Part model, mm, in its own coordinate system. Face numbers are marked on the shaded views. Give positions to 0.01 mm unless a question says otherwise; leave off trailing zeros. Write each loop counter-clockwise with the first axis right and the second up, starting at its lowest first coordinate (ties: lowest second). Pieces come first, ordered by that corner, then holes.
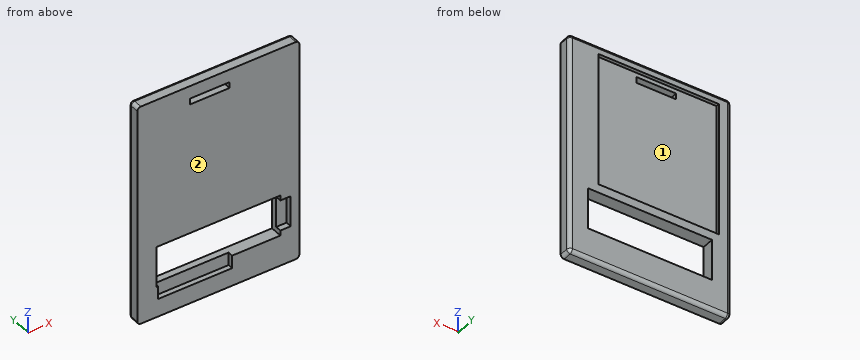
```python
from build123d import *

# Parameters (mm, degrees)
SKETCH1_W           = 94
SKETCH1_H           = 130
BOSS_EXTRUDE1_DEPTH = 7
SKETCH2_W           = 72
SKETCH2_H           = 24
CUT_EXTRUDE1_DEPTH  = 8
SKETCH3_W           = 6
SKETCH3_H           = 18
CUT_EXTRUDE2_DEPTH  = 3.5
SKETCH4_W           = 43
SKETCH4_H           = 7.5
CUT_EXTRUDE3_DEPTH  = 3
SKETCH5_W           = 70
SKETCH5_H           = 78
CUT_EXTRUDE4_DEPTH  = 2
SKETCH6_W           = 23
SKETCH6_H           = 3.5
CUT_EXTRUDE5_DEPTH  = 6
FILLET1_R           = 2


with BuildPart() as part:
    # Sketch1 → Boss-Extrude1 (new body)
    with BuildSketch(Plane(origin=(0, 0, 0), x_dir=(1, 0, 0), z_dir=(0, 1, 0))):
        with Locations((47, 65)):
            Rectangle(SKETCH1_W, SKETCH1_H)
    extrude(amount=BOSS_EXTRUDE1_DEPTH)

    # Sketch2 → Cut-Extrude1 (cut, through all)
    with BuildSketch(Plane(origin=(0, 7, 0), x_dir=(1, 0, 0), z_dir=(0, 1, 0))):
        with Locations((47, 100)):
            Rectangle(SKETCH2_W, SKETCH2_H)
    extrude(amount=-CUT_EXTRUDE1_DEPTH, mode=Mode.SUBTRACT)

    # Sketch3 → Cut-Extrude2 (cut)
    with BuildSketch(Plane.XZ):
        with Locations((86, -100)):
            Rectangle(SKETCH3_W, SKETCH3_H)
    extrude(amount=-CUT_EXTRUDE2_DEPTH, mode=Mode.SUBTRACT)

    # Sketch4 → Cut-Extrude3 (cut)
    with BuildSketch(Plane.XZ):
        with Locations((33.5, -115.75)):
            Rectangle(SKETCH4_W, SKETCH4_H)
    extrude(amount=-CUT_EXTRUDE3_DEPTH, mode=Mode.SUBTRACT)

    # Sketch5 → Cut-Extrude4 (cut)
    with BuildSketch(Plane(origin=(0, 7, 0), x_dir=(1, 0, 0), z_dir=(0, 1, 0))):
        with Locations((42, 44)):
            Rectangle(SKETCH5_W, SKETCH5_H)
    extrude(amount=-CUT_EXTRUDE4_DEPTH, mode=Mode.SUBTRACT)

    # Sketch6 → Cut-Extrude5 (cut, through all)
    with BuildSketch(Plane(origin=(0, 5, 0), x_dir=(1, 0, 0), z_dir=(0, 1, 0))):
        with Locations((42, 9.25)):
            Rectangle(SKETCH6_W, SKETCH6_H)
    extrude(amount=-CUT_EXTRUDE5_DEPTH, mode=Mode.SUBTRACT)

    # Fillet1
    fillet1_edges = [part.edges().sort_by_distance(p)[0] for p in [
        (94, 7, -65),
        (47, 7, -130),
        (0, 7, -65),
        (0, 3.5, -130),
        (94, 3.5, -130),
        (94, 3.5, 0),
        (0, 3.5, 0),
        (47, 7, 0),
    ]]
    fillet(fillet1_edges, radius=FILLET1_R)


solid = part.part
```
1) Saw through at B-B, the plane z = -46. Write the cut outline in (x, y), then the cut area to 3 significant figures.
Answers follow:
outline: (0, 0) - (94, 0) - (94, 5) arc R2 ccw to (92, 7) - (77, 7) - (77, 5) - (7, 5) - (7, 7) - (2, 7) arc R2 ccw to (0, 5) - close
area: 516 mm2
2) Pin check, flat tips, straight feed: pin 1 Ø8 at (x, z) = (33, -114) entering from -Y; pin 2 Ø1.5 at (y, z) = (6, -20) entering from +X; pin 3 Ø1.6 at (y, z) = (6, -48.5) entering from -X; pin 4 Ø5 at (x, z) = (87, -97) entering from -Y. Stop position of each tip, or through.
Answers follow:
pin 1: stops at y = 3
pin 2: stops at x = 93.98
pin 3: stops at x = 0.01
pin 4: stops at y = 0
3) Saw through at C-C, the plane x = 86. Write the cut outline in (y, z), then the cut area to 3 significant figures.
Answers follow:
outline: (0, -130) - (5, -130) arc R2 ccw to (7, -128) - (7, -2) arc R2 ccw to (5, 0) - (0, 0) - (0, -91) - (3.5, -91) - (3.5, -109) - (0, -109) - close
area: 845 mm2
4) Saw through at A-A, the plane x = 33. Write the cut outline in (y, z), then the cut area to 3 significant figures.
Answers follow:
outline: (0, -130) - (5, -130) arc R2 ccw to (7, -128) - (7, -112) - (3, -112) - (3, -119.5) - (0, -119.5) - close; (0, -88) - (7, -88) - (7, -83) - (5, -83) - (5, -11) - (0, -11) - close; (0, -7.5) - (5, -7.5) - (5, -5) - (7, -5) - (7, -2) arc R2 ccw to (5, 0) - (0, 0) - close
area: 544 mm2
5) Saw through at D-D, the plane y = 1.25. Write the cut outline in (x, z), then the cut area to 3 significant figures.
Answers follow:
outline: (0, -128) arc R2 ccw to (2, -130) - (92, -130) arc R2 ccw to (94, -128) - (94, -2) arc R2 ccw to (92, 0) - (2, 0) arc R2 ccw to (0, -2) - close; hole (11, -112) - (12, -112) - (12, -119.5) - (55, -119.5) - (55, -112) - (83, -112) - (83, -109) - (89, -109) - (89, -91) - (83, -91) - (83, -88) - (11, -88) - close; hole (30.5, -11) - (53.5, -11) - (53.5, -7.5) - (30.5, -7.5) - close
area: 9,980 mm2
6) Wall check: L1, parallel to Z at x = 66, y = 1.75; L2, parallel to Z at x = 36, y = 4; L3, parallel to Z at x = 15, y = 6.75. Give the ranges that are in metal, low to high.
Answers follow:
L1: z = -130 to -112, -88 to 0
L2: z = -130 to -112, -88 to -11, -7.5 to 0
L3: z = -128.97 to -112, -88 to -83, -5 to -1.03
7) Two-plate mould, pull along X, no slides. Class the marked faces 1 and 2: +X half, -X half, draft (parallel to the pull), parting line (faces both ways), or undercut.
Answers follow:
face 1: undercut
face 2: draft
